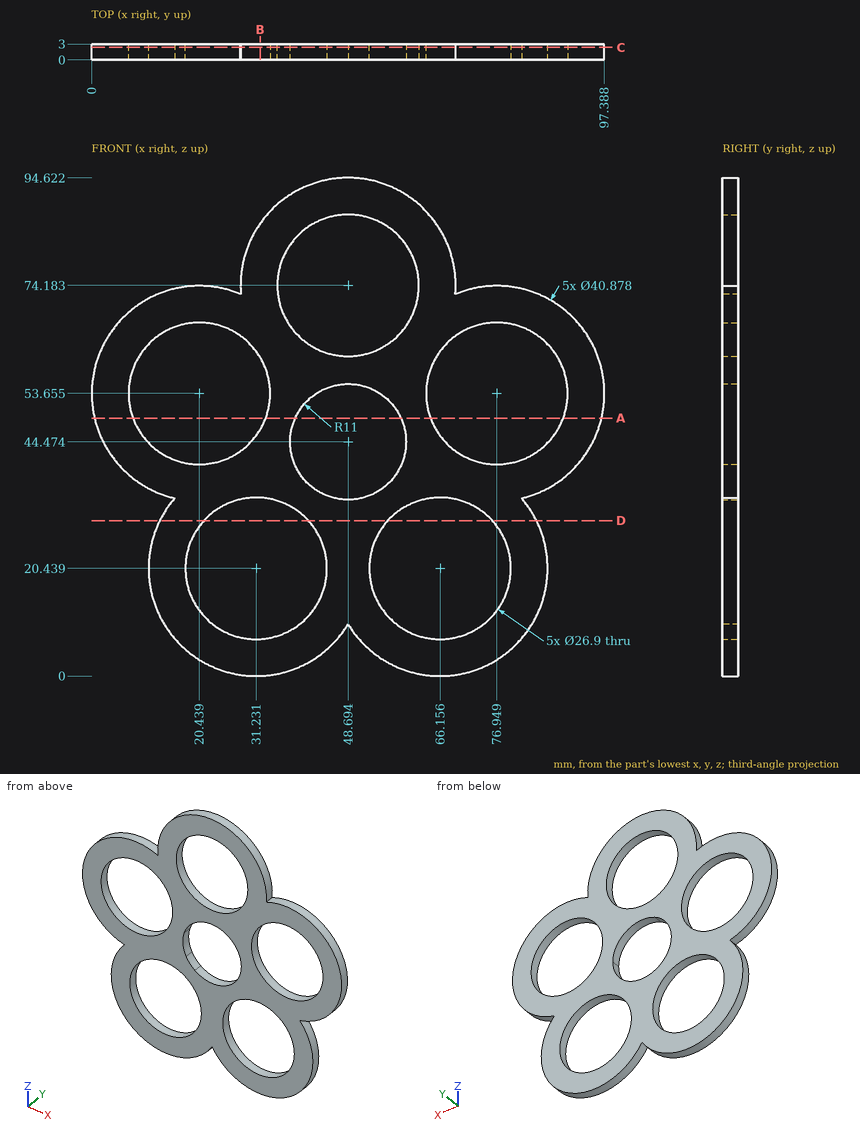
Could you check a few things on this drawing? It's one solid part, dimensions in mm from its lowest x, y, z. Coordinates: 2 decimals unless noted, no trailing zeros. Write each loop counter-clockwise with the first axis right and the second up, starting at its lowest first coordinate (ties: lowest second). Pieces come first, ordered by that corner, then holes.
Q1. Imagine slicing it at D-D, the plane z = 29.5. List the corners of the cut face in (x, y) for me.
Results found:
outline: (12.91, 0) - (21.29, 0) - (21.29, 3) - (12.91, 3) - close; (41.17, 0) - (56.22, 0) - (56.22, 3) - (41.17, 3) - close; (76.1, 0) - (84.48, 0) - (84.48, 3) - (76.1, 3) - close
Q2. Imagine slicing it at A-A, the plane z = 49. List the corners of the cut face in (x, y) for me.
Results found:
outline: (0.54, 0) - (7.82, 0) - (7.82, 3) - (0.54, 3) - close; (33.06, 0) - (38.67, 0) - (38.67, 3) - (33.06, 3) - close; (58.72, 0) - (64.33, 0) - (64.33, 3) - (58.72, 3) - close; (89.57, 0) - (96.85, 0) - (96.85, 3) - (89.57, 3) - close
Q3. Imagine slicing it at C-C, the plane y = 2.35. Count the separate pieces of the cut face and the enclosed holes in it, plus the area to 3 significant figures.
Results found:
separate pieces: 1
enclosed holes: 6
area: 3,260 mm2
Q4. Imagine slicing it at B-B, the plane x = 32. List the corners of the cut face in (y, z) for me (1 decimal).
Results found:
outline: (0, 0) - (3, 0) - (3, 7) - (0, 7) - close; (0, 33.9) - (3, 33.9) - (3, 46.8) - (0, 46.8) - close; (0, 60.5) - (3, 60.5) - (3, 86) - (0, 86) - close
Q5. For P1, Ø16, axis at x = 48.69, z = 74.18, coming from the +Y side, with a flat end and sliding along its axis, tell me the tip position at first contact or that it passes through.
Results found:
P1: passes through
Q6. Please list where these lines run through material, in increasing order: L1, parallel to X at y = 2.1, z = 58; L2, parallel to X at y = 2.6, z = 54 (1 decimal); L3, parallel to X at y = 1.9, z = 30 (1 decimal).
Results found:
L1: x = 0.47 to 7.71, 33.17 to 64.22, 89.68 to 96.92
L2: x = 0 to 7, 33.9 to 43.2, 54.2 to 63.5, 90.4 to 97.4
L3: x = 13.2 to 21.8, 40.7 to 56.7, 75.6 to 84.2
